Study the drawing (mm; zero at the part's minimum x, y, z) and answer. Give positions to 0.01 mm unless a question says otherwise; leave off trailing zeros. Order: outer loops, then holes, each group sorted by start corner. A loop starts at its lowest first (then second) coordinate and runs counter-clockwise, first axis right, second up. Notation, with made-up numbers: (-8, 35) -> (5, 35) arc R12 cw to (5, 47) -> close; hole circle Ø2 at (71.5, -36.5). An arc over 180 degrees is marked (long way). Use a Markdown table: item, result. Add a question column.
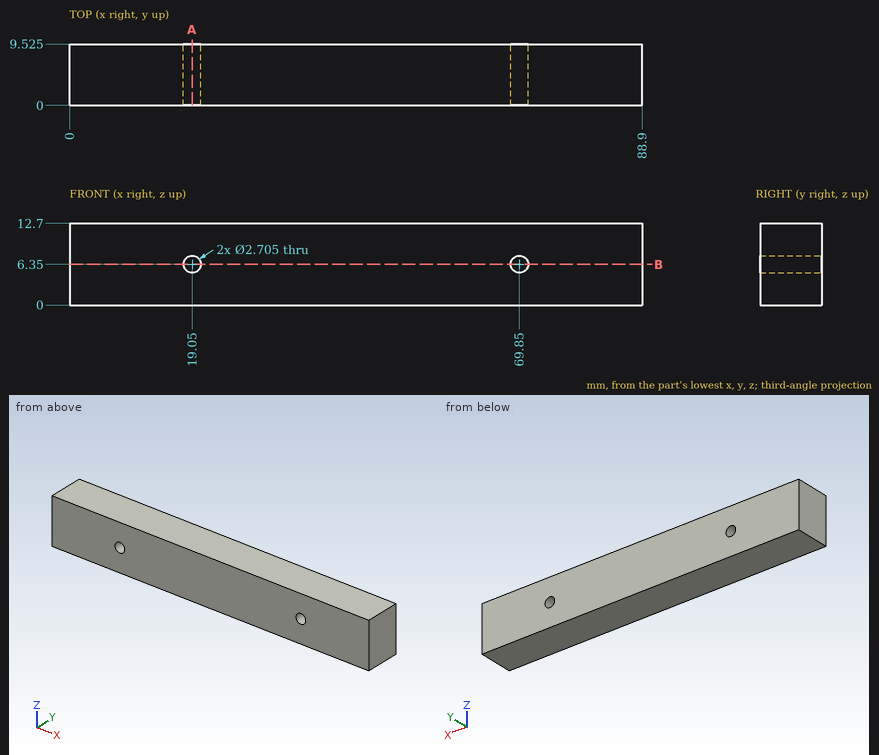
1) Straight lines are drawn through the part: line 1 (X direction, y = 5.5, z = 6.5); line 2 (Z direction, x = 19.05, y = 2.75); line 3 (X direction, y = 6.75, z = 5.75). For each, find the intervals that lie inside material, in ascending order.
2) Flat-ended cylindrical pins translate along their axes: pin 1 (2 mm diameter, centred on y = 7.5, z = 6.5, fed in from -X); pin 2 (1.6 mm diameter, centred on x = 19.05, z = 6.35, fed in from +Y). Find the tip coordinate at first contact, or state that the pin passes through.
3) The part is cut by section B-B, the plane z = 6.35. Determine the outline of the cut face in (x, y) (1 decimal).
4) The part is cut by section A-A, the plane x = 19.05. Determine the outline of the cut face in (y, z) (1 decimal).
A:
| question | item | result |
|---|---|---|
| 1 | line 1 | 0 to 17.71, 20.39 to 68.51, 71.19 to 88.9 |
| 1 | line 2 | 0 to 5, 7.7 to 12.7 |
| 1 | line 3 | 0 to 17.84, 20.26 to 68.64, 71.06 to 88.9 |
| 2 | pin 1 | x = 0 |
| 2 | pin 2 | through |
| 3 | outline | (0, 0) -> (17.7, 0) -> (17.7, 9.5) -> (0, 9.5) -> close; (20.4, 0) -> (68.5, 0) -> (68.5, 9.5) -> (20.4, 9.5) -> close; (71.2, 0) -> (88.9, 0) -> (88.9, 9.5) -> (71.2, 9.5) -> close |
| 4 | outline | (0, 0) -> (9.5, 0) -> (9.5, 5) -> (0, 5) -> close; (0, 7.7) -> (9.5, 7.7) -> (9.5, 12.7) -> (0, 12.7) -> close |
